Geometry check sheet. Reference: the model listing, model coordinates, mm. Face numbers are marked on the shaded views. A direction names the side the tool comes from. Give positions to 0.01 mm unless a question says otherwise; leave off trailing zeros. Order: outer loops, then holes, each group sorted by start corner. A loop starts at its lowest first (then second) coordinate and runs counter-clockwise, first axis right, second up. Notation, with made-up numbers: M 56.5,7 L 65.5,7 A24 ccw 65.5,17 Z; hole C 88,-22.75 d8. An arc over 180 degrees is marked long. Answer as CSV lines item,"result".
from build123d import *

# Parameters (mm, degrees)
SKETCH1_W           = 21
SKETCH1_H           = 40
BOSS_EXTRUDE1_DEPTH = 45
SKETCH2_W           = 21
SKETCH2_H           = 3
BOSS_EXTRUDE2_DEPTH = 7.5
SKETCH3_W           = 21
SKETCH3_H           = 3
BOSS_EXTRUDE3_DEPTH = 7.5
SKETCH5_R           = 3
BOSS_EXTRUDE4_DEPTH = 4


with BuildPart() as part:
    # Sketch1 → Boss-Extrude1 (new body)
    with BuildSketch(Plane(origin=(0, 0, 0), x_dir=(1, 0, 0), z_dir=(0, 1, 0))):
        Rectangle(SKETCH1_W, SKETCH1_H)
    extrude(amount=BOSS_EXTRUDE1_DEPTH)

    # Sketch2 → Boss-Extrude2 (add)
    with BuildSketch(Plane.XY.offset(20)):
        with Locations((0, 34.5)):
            Rectangle(SKETCH2_W, SKETCH2_H)
    extrude(amount=BOSS_EXTRUDE2_DEPTH)

    # Sketch3 → Boss-Extrude3 (add)
    with BuildSketch(Plane(origin=(0, 0, -20), x_dir=(-1, 0, 0), z_dir=(0, 0, -1))):
        with Locations((0, 34.5)):
            Rectangle(SKETCH3_W, SKETCH3_H)
    extrude(amount=BOSS_EXTRUDE3_DEPTH)

    # Sketch5 → Boss-Extrude4 (add)
    with BuildSketch(Plane(origin=(0, 45, 0), x_dir=(1, 0, 0), z_dir=(0, 1, 0))):
        with Locations(Location((0, -13.620158604, 0), (0, 0, 90))):
            Circle(SKETCH5_R)
    extrude(amount=BOSS_EXTRUDE4_DEPTH)


solid = part.part
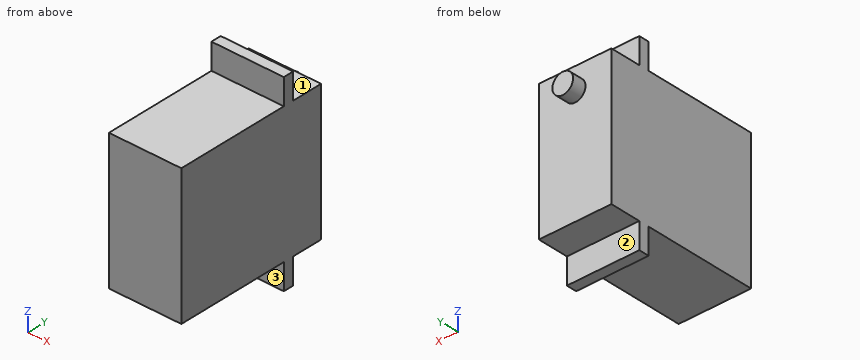
(1) Gauge pin test, flat ends, axial feed: P1, Ø6, axis at x = 2, z = 24.5, coming from the -Y side; P2, Ø8, axis at x = 5, y = 30, coming from the +Z side; P3, Ø4.5, axis at x = 0.5, y = 39.5, coming from the +Z side; P4, Ø10, axis at x = 4.5, y = 42.5, coming from the -Z side. Record the tip position at first contact, or that the pin passes through.
The answers:
P1,"stops at y = 33"
P2,"stops at z = 27.5"
P3,"stops at z = 20"
P4,"stops at z = -20"
(2) Material ranges on line 1 (Y direction, x = 0.25, z = 22); line 2 (Y direction, x = 8.5, z = -12.5); line 3 (Z direction, x = 1, y = 25.5), recorded low to high.
The answers:
line 1,"y = 33 to 36"
line 2,"y = 0 to 45"
line 3,"z = -20 to 20"
(3) Section check D-D on x = -8.25. Enter the section's corners in (y, z).
The answers:
outline,"M 0,-20 L 33,-20 L 33,-27.5 L 36,-27.5 L 36,-20 L 45,-20 L 45,20 L 36,20 L 36,27.5 L 33,27.5 L 33,20 L 0,20 Z"
(4) Section check B-B on z = 16. Enter the section's corners in (x, y), then the cut area to 3 significant figures.
The answers:
outline,"M -10.5,0 L 10.5,0 L 10.5,45 L 1.83,45 L 1.83,49 L -1.83,49 L -1.83,45 L -10.5,45 Z"
area,"960 mm2"
(5) Section check C-C on y = 12.5. Enter the section's corners in (x, z), then the cut area to 3 significant figures.
The answers:
outline,"M -10.5,-20 L 10.5,-20 L 10.5,20 L -10.5,20 Z"
area,"840 mm2"
(6) Tool access check on the marked faces 1, 2 and 3. Record the directions out of +Z, -Z, +X, -X, +Y, -Y that give a thin tool (end or side, any length) a straight path to the whole face; none if there is none.
The answers:
face 1,"+Z, +X, -X, +Y"
face 2,"-Z, +X, -X, +Y"
face 3,"-Z, +X, -X, -Y"
(7) Section check A-A on x = 0. Enter the section's corners in (y, z).
The answers:
outline,"M 0,-20 L 33,-20 L 33,-27.5 L 36,-27.5 L 36,-20 L 45,-20 L 45,10.62 L 49,10.62 L 49,16.62 L 45,16.62 L 45,20 L 36,20 L 36,27.5 L 33,27.5 L 33,20 L 0,20 Z"
